Here's how the part is built. I have some questions about the finished solid (model axes, mm). A direction names the side the tool comes from. Give positions to 0.01 mm unless a question says otherwise; leave off trailing zeros. Write each loop counter-clockwise with the first axis right and the second up, starting at its lowest first coordinate (ties: lowest second). Pieces come first, ordered by that corner, then holes. Notation, with made-up numbers: (59.5, 51.25) - (112.5, 51.25) arc R30 ccw to (112.5, 82.25) - close; hole circle Ø11 at (50, 79.5). An arc over 180 degrees is marked (long way). Use a Markdown table: item, result.
```python
from build123d import *

# Parameters (mm, degrees)
CROQUIS1_R              = 4
SALIENTE_EXTRUIR1_DEPTH = 230


with BuildPart() as part:
    # Croquis1 → Saliente-Extruir1 (new body)
    with BuildSketch(Plane(origin=(0, 0, 0), x_dir=(1, 0, 0), z_dir=(0, 1, 0))):
        with BuildLine():
            Line((-7, 15), (-15, 15))
            Line((-15, 15), (-15, 5.027604917))
            Line((-15, 5.027604917), (-12.623437069, 5.027604917))
            Line((-12.623437069, 5.027604917), (-12.623437069, 7.752682341))
            Line((-12.623437069, 7.752682341), (-11.320548438, 7.752682341))
            Line((-11.320548438, 7.752682341), (-7, 3.432133903))
            Line((-7, 3.432133903), (-7, -2.861090311))
            Line((-7, -2.861090311), (-12.793007796, -7))
            Line((-12.793007796, -7), (-13.527286117, -7))
            Line((-13.527286117, -7), (-13.527286117, -1.25796789))
            Line((-13.527286117, -1.25796789), (-15, -1.25796789))
            Line((-15, -1.25796789), (-15, -15))
            Line((-15, -15), (-3.139941254, -15))
            Line((-3.139941254, -15), (-3.139941254, -12.505835019))
            Line((-3.139941254, -12.505835019), (-6.77895709, -12.505835019))
            Line((-6.77895709, -12.505835019), (-6.77895709, -10.079824462))
            Line((-6.77895709, -10.079824462), (-2.512909638, -7.031876702))
            Line((-2.512909638, -7.031876702), (3.25590476, -7.031876702))
            Line((3.25590476, -7.031876702), (6.894920596, -10.079824462))
            Line((6.894920596, -10.079824462), (6.894920596, -12.505835019))
            Line((6.894920596, -12.505835019), (3.25590476, -12.505835019))
            Line((3.25590476, -12.505835019), (3.25590476, -15))
            Line((3.25590476, -15), (15, -15))
            Line((15, -15), (15, -7))
            ThreePointArc((15, -7), (8.556349186, 8.556349186), (-7, 15))
        make_face()
        Circle(CROQUIS1_R, mode=Mode.SUBTRACT)
    extrude(amount=SALIENTE_EXTRUIR1_DEPTH)


solid = part.part
```
Item 1: Will these pins go through, and if not, where does the flat tip stop? pin 1 Ø4 at (x, y) = (6, 96.5) entering from -Z; pin 2 Ø1.7 at (y, z) = (141, 3) entering from +X; pin 3 Ø0.8 at (y, z) = (142, -6.5) entering from +X; pin 4 Ø4 at (x, z) = (-0.5, 1) entering from -Y (3 decimals).
Values:
| item | result |
|---|---|
| pin 1 | stops at z = -12.05 |
| pin 2 | stops at x = 14.77 |
| pin 3 | stops at x = 10.67 |
| pin 4 | passes through |
Item 2: If we section it at C-C, the plane z = -13: Write out the boundary of the cut face in (x, y), plus the area to 3 significant figures.
Values:
| item | result |
|---|---|
| outline | (-15, 0) - (2.17, 0) - (2.17, 230) - (-15, 230) - close |
| area | 3,950 mm2 |
Item 3: Thinking about a two-plate mould opening in Z: for faces 4 (the flat face through (-11, 113, -15)), 5 (the flat face through (-5, 113, 12.506)), 6 (the flat face through (5.05, 113.39, 8.535)), 7 (the flat face through (-4, 230, 3)), which applies, +Z half, -Z half, draft (parallel to the pull), parting line (faces both ways), or undercut?
Values:
| item | result |
|---|---|
| face 4 | -Z half |
| face 5 | undercut |
| face 6 | undercut |
| face 7 | draft |
Item 4: I need wall thicknesses on line 1 along X through (y, z) = (74, 12); line 2 along Z through (x, y) = (-13, 60.5); line 3 along X through (y, z) = (156.5, 0). Which ranges of each line are inside material? Lowest first, please. Write a range as [from, to].
Values:
| item | result |
|---|---|
| line 1 | x = [-15, -6.78], [6.89, 15] |
| line 2 | z = [-15, -5.03], [7, 15] |
| line 3 | x = [-7, -4], [4, 13.86] |
Item 5: If we section it at B-B, the plane x = 0: Write out the boundary of the cut face in (y, z).
Values:
| item | result |
|---|---|
| outline | (0, -13.86) - (230, -13.86) - (230, -4) - (0, -4) - close; (0, 4) - (230, 4) - (230, 7.03) - (0, 7.03) - close |
Item 6: If we section it at A-A, the plane y = 175.5: Write out the boundary of the cut face in (x, z), plus the area to 3 significant figures.
Values:
| item | result |
|---|---|
| outline | (-15, -15) - (-7, -15) arc R22 ccw to (15, 7) - (15, 15) - (3.26, 15) - (3.26, 12.51) - (6.89, 12.51) - (6.89, 10.08) - (3.26, 7.03) - (-2.51, 7.03) - (-6.78, 10.08) - (-6.78, 12.51) - (-3.14, 12.51) - (-3.14, 15) - (-15, 15) - (-15, 1.26) - (-13.53, 1.26) - (-13.53, 7) - (-12.79, 7) - (-7, 2.86) - (-7, -3.43) - (-11.32, -7.75) - (-12.62, -7.75) - (-12.62, -5.03) - (-15, -5.03) - close; hole circle Ø8 at (0, 0) |
| area | 585 mm2 |
Item 7: For faces 1 (the flat face through (0, 113, 7.032)), 2 (the flat face through (-9.19, 113.39, -5.62)), 3 (the flat face through (-15, 113, -10)), which set-ups out of +Z, -Z, +X, -X, +Y, -Y let a thin tool reach every point of the face, with its end or its side?
Values:
| item | result |
|---|---|
| face 1 | +Z, +Y, -Y |
| face 2 | +Y, -Y |
| face 3 | +Z, -Z, -X, +Y, -Y |
